Design review of the part built by this model. Coordinates are the model's own, in mm. Face numbers are marked on the shaded views. Coordinates: 2 decimals unless noted, no trailing zeros. Order: outer loops, then holes, each group sorted by start corner. A loop starts at its lowest first (then second) coordinate and runs counter-clockwise, first axis right, second up. Notation, with made-up numbers: M 18.25,57.25 L 45.25,57.25 A26 cw 45.25,73.25 Z; hole C -38.5,-7 d9. An arc over 180 degrees is marked long. Answer as a JSON object with one key per item and string values.
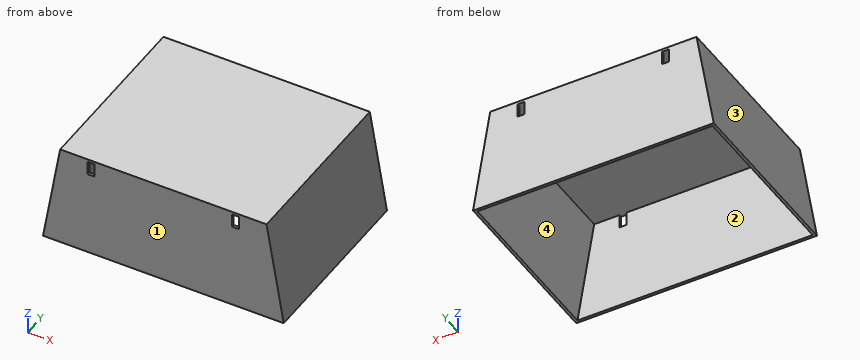
from build123d import *

# Parameters (mm, degrees)
EXTRUDE_2_DEPTH     = 130
SHELL_2_T           = -4
SKETCH_5_W          = 10
SKETCH_5_H          = 20
CUT_EXTRUDE_1_DEPTH = 260


with BuildPart() as part:
    # 草图1 → 凸台-拉伸2 (new, symmetric)
    with BuildSketch(Plane(origin=(0, 0, 0), x_dir=(1, 0, 0), z_dir=(0, 1, 0))):
        Polygon((175, 0), (-175, 0), (-150, -150), (150, -150), align=None)
    extrude(amount=EXTRUDE_2_DEPTH, both=True)

    # 抽壳2
    shell_2_openings = [part.faces().sort_by_distance(p)[0] for p in [
        (0, 0, 0),
    ]]
    offset(amount=SHELL_2_T, openings=shell_2_openings, kind=Kind.INTERSECTION)

    # 草图5 → 切除-拉伸1 (cut)
    with BuildSketch(Plane(origin=(0, 130, 0), x_dir=(1, 0, 0), z_dir=(0, 1, 0))):
        with Locations((-105, -136)):
            Rectangle(SKETCH_5_W, SKETCH_5_H)
        with Locations((105, -136)):
            Rectangle(SKETCH_5_W, SKETCH_5_H)
    extrude(amount=-CUT_EXTRUDE_1_DEPTH, mode=Mode.SUBTRACT)


solid = part.part
1) To check wall thickness, follow L1, parallel to Y at x = -58, z = 135.5; L2, parallel to Z at x = -88, y = 85.5; L3, parallel to X at y = -47, z = 123.5. State the ranges of each line that lie inside material, in increasing order.
Taken from the geometry:
{"L1": "y = -130 to -126, 126 to 130", "L2": "z = 146 to 150", "L3": "x = -154.42 to -150.36, 150.36 to 154.42"}
2) Add section A-A (x = 63.5). State the section outline as (y, z) points, and give its area (3 significant figures).
Taken from the geometry:
{"outline": "M -130,0 L -126,0 L -126,146 L 126,146 L 126,0 L 130,0 L 130,150 L -130,150 Z", "area": "2,210 mm2"}
3) Add section C-C (y = 70). State the section outline as (x, z) points, and give its area (3 significant figures).
Taken from the geometry:
{"outline": "M -175,0 L -170.94,0 L -146.61,146 L 146.61,146 L 170.94,0 L 175,0 L 150,150 L -150,150 Z", "area": "2,390 mm2"}
4) Insertion check: pin 1 Ø4 at (y, z) = (-5.5, 28.5) entering from +X; pin 2 Ø4.5 at (y, z) = (-128.5, 133.5) entering from -X (3 decimals); pin 3 Ø8 at (x, y) = (-53.5, 103.5) entering from -Z. Each pin has a flat end and moves straight along its axis. Give the tip position at first contact, or say it passes through.
Taken from the geometry:
{"pin 1": "stops at x = 170.58", "pin 2": "stops at x = -153.125", "pin 3": "stops at z = 146"}
5) Mouldability with a two-part tool opening along X and no side actions: class the marked faces 1, 2, 3 and 4 as released by +X, released by -X, zero draft, split by the parting line, or undercut.
Taken from the geometry:
{"face 1": "zero draft", "face 2": "undercut", "face 3": "released by -X", "face 4": "undercut"}
6) Add section B-B (z = 48). State the section outline as (x, y) points, and give its area (3 significant figures).
Taken from the geometry:
{"outline": "M -167,-130 L 167,-130 L 167,130 L -167,130 Z; hole M -162.94,-126 L 162.94,-126 L 162.94,126 L -162.94,126 Z", "area": "4,720 mm2"}
7) Add section D-D (z = 74). State the section outline as (x, y) points.
Taken from the geometry:
{"outline": "M -162.67,-130 L 162.67,-130 L 162.67,130 L -162.67,130 Z; hole M -158.61,-126 L 158.61,-126 L 158.61,126 L -158.61,126 Z"}
